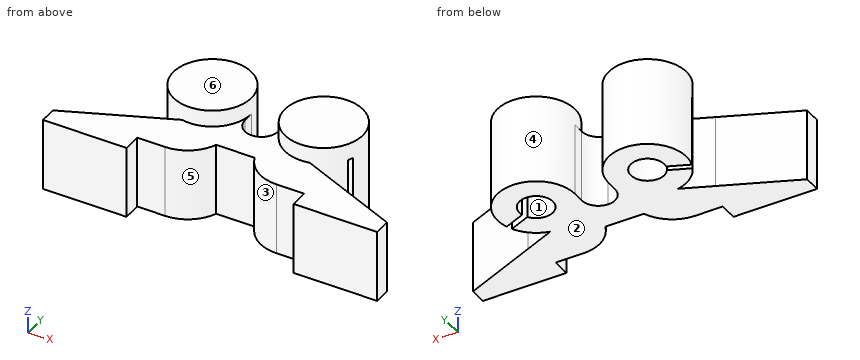
from build123d import *

# Parameters (mm, degrees)
SKETCH1_R           = 7
BOSS_EXTRUDE1_DEPTH = 13
SKETCH2_R           = 7
BOSS_EXTRUDE2_DEPTH = 3
SKETCH3_R           = 3
CUT_EXTRUDE1_DEPTH  = 13


with BuildPart() as part:
    # Sketch1 → Boss-Extrude1 (new body)
    with BuildSketch(Plane.XY):
        with Locations((10, 0)):
            Circle(SKETCH1_R)
        with BuildLine():
            ThreePointArc((3.461651585, -10), (6.031373033, -13.266281297), (10, -14.5))
            Line((10, -14.5), (15, -14.5))
            Line((15, -14.5), (15, -17.75))
            Line((15, -17.75), (30, -17.75))
            Line((30, -17.75), (30, -14.75))
            Line((30, -14.75), (16.808917195, -9.124391157))
            Line((16.808917195, -9.124391157), (11.464397441, -6.845110674))
            ThreePointArc((11.464397441, -6.845110674), (5.598340205, -5.442921187), (3, 0))
            Line((3, 0), (3, -2))
            ThreePointArc((3, -2), (2.121320344, -4.121320344), (0, -5))
            Line((0, -5), (0, -10))
            Line((0, -10), (3.461651585, -10))
        make_face()
    extrude(amount=BOSS_EXTRUDE1_DEPTH)

    # Sketch2 → Boss-Extrude2 (add)
    with BuildSketch(Plane.XY.offset(13)):
        with Locations(Location((10, 0, 0), (0, 0, 180))):
            Circle(SKETCH2_R)
    extrude(amount=BOSS_EXTRUDE2_DEPTH)

    # Sketch3 → Cut-Extrude1 (cut)
    with BuildSketch(Plane.XY):
        with Locations((10, 0)):
            Circle(SKETCH3_R)
        with BuildLine():
            ThreePointArc((12.917076099, -0.70047629), (12.759529774, -1.176858286), (12.524790004, -1.620319548))
            Line((12.524790004, -1.620319548), (16.664084665, -3.385606977))
            Line((16.664084665, -3.385606977), (17.05637076, -2.465763719))
            Line((17.05637076, -2.465763719), (12.917076099, -0.70047629))
        make_face()
    extrude(amount=CUT_EXTRUDE1_DEPTH, mode=Mode.SUBTRACT)

    # Mirror1: part across plane


with BuildPart() as part_1:
    add(part.part)
    add(part.part.mirror(Plane(origin=(0, 0, 0), x_dir=(0, 0, 1), z_dir=(1, 0, 0))))


solid = part_1.part
Here's how the part is built. I have some questions about the finished solid (model axes, mm). Face numbers are marked on the shaded views. A direction names the side the tool comes from. Round coordinates to 2 decimals unless told otherwise and drop trailing zeros. Order: outer loops, then holes, each group sorted by start corner. A loop starts at its lowest first (then second) coordinate and runs counter-clockwise, first axis right, second up. Notation, with made-up numbers: (23, 8.5) -> (66, 8.5) arc R34 cw to (66, 39.5) -> close; hole circle Ø4 at (69, -35.75). An arc over 180 degrees is marked (long way). Return JSON: item names as keys, results as strings.
Q1. If we mould it in two halves opening along Y, with no side actions, what happens to the marked faces 4, 5 and 6? For each: released by +Y, released by -Y, zero draft, split by the parting line, or undercut.
Filled sheet:
{"face 4": "undercut", "face 5": "released by -Y", "face 6": "zero draft"}
Q2. If we section it at B-B on z = 4: List the corners of the cut face in (x, y) for me.
Filled sheet:
{"outline": "(-30, -17.75) -> (-15, -17.75) -> (-15, -14.5) -> (-10, -14.5) arc R7 ccw to (-3.46, -10) -> (3.46, -10) arc R7 ccw to (10, -14.5) -> (15, -14.5) -> (15, -17.75) -> (30, -17.75) -> (30, -14.75) -> (11.46, -6.85) arc R7 ccw to (16.23, -3.2) -> (12.52, -1.62) arc R3 cw (long way) to (12.92, -0.7) -> (16.62, -2.28) arc R7 ccw (long way) to (3, 0) -> (3, -2) arc R3 cw to (-3, -2) -> (-3, 0) arc R7 ccw (long way) to (-16.62, -2.28) -> (-12.92, -0.7) arc R3 cw (long way) to (-12.52, -1.62) -> (-16.23, -3.2) arc R7 ccw to (-11.46, -6.85) -> (-30, -14.75) -> close"}
Q3. Which directions (+Z, -Z, +X, -X, +Y, -Y) give clear straight access to the entire face, cutting with the end or side of a thin tool? Please do the marked faces 1, 2 and 3.
Filled sheet:
{"face 1": "-Z", "face 2": "-Z, +X, -X, +Y, -Y", "face 3": "+Z, -Z, -Y"}
Q4. If we section it at D-D on y = 5.25: List the corners of the cut face in (x, z) for me, plus the area to 3 significant figures.
Filled sheet:
{"outline": "(-14.63, 0) -> (-5.37, 0) -> (-5.37, 16) -> (-14.63, 16) -> close; (5.37, 0) -> (14.63, 0) -> (14.63, 16) -> (5.37, 16) -> close", "area": "296 mm^2"}
Q5. I need wall thicknesses on line 1 along X through (y, z) = (0, 6); line 2 along X through (y, z) = (-1.25, 7.5); line 3 along X through (y, z) = (-2, 8). Which ranges of each line are inside material? Lowest first, please. Write a range as from..to.
Filled sheet:
{"line 1": "x = -17..-13, -7..-3, 3..7, 13..17", "line 2": "x = -16.89..-14.21, -7.27..-3, 3..7.27, 14.21..16.89", "line 3": "x = -16.71..-15.96, -13.42..-12.24, -7.76..-3, 3..7.76, 12.24..13.42, 15.96..16.71"}
Q6. If we section it at C-C on z = 14.25: List the corners of the cut face in (x, y) for me.
Filled sheet:
{"outline": "circle Ø14 at (-10, 0); circle Ø14 at (10, 0)"}
Q7. For pin 1 Ø5 at (x, y) = (10, 0) entering from -Z; pin 2 Ø8 at (y, z) = (-6, 12) entering from -X; pin 3 Ø1.6 at (y, z) = (-1.5, 3.5) entering from +X; pin 4 Ø5 at (x, y) = (-19.5, 3.5) entering from -Z, each with a flat end and sliding along its axis, tell me the tip position at first contact or that it passes through.
Filled sheet:
{"pin 1": "stops at z = 13", "pin 2": "stops at x = -18.86", "pin 3": "stops at x = 16.96", "pin 4": "passes through"}
Q8. If we section it at A-A on y = -11: List the corners of the cut face in (x, z) for me.
Filled sheet:
{"outline": "(-21.21, 0) -> (-3.94, 0) -> (-3.94, 13) -> (-21.21, 13) -> close; (3.94, 0) -> (21.21, 0) -> (21.21, 13) -> (3.94, 13) -> close"}
